from build123d import *

# Parameters (mm, degrees)
F0_W        = 15
F0_H        = 15
F0_W_2      = 7
F0_H_2      = 7
F1_DEPTH    = 4
F2_W        = 7
F2_H        = 7
F3_DEPTH    = 4
F3_TAPER    = 5
F4_W        = 7
F4_H        = 4
F5_DEPTH    = 25
F6_W        = 7
F6_H        = 4
F7_DEPTH    = 25
F8_T1_DEPTH = 37.1662479036
F9_R        = 2.5


# Not quite as in the source:
# - a fillet or chamfer that OpenCascade refuses, or shapes differently, is made with other operations: its cross-section is extruded or revolved along the edge and cut away or added


with BuildPart() as f1:
    # F0 (on Top) → F1 (new body)
    with BuildSketch(Plane.XY):
        Rectangle(F0_W, F0_H)
        Rectangle(F0_W_2, F0_H_2, mode=Mode.SUBTRACT)
        Rectangle(F0_W_2, F0_H_2)
    extrude(amount=F1_DEPTH)

    # F2 (on face) → F3 (cut)
    with BuildSketch(Plane.XY.offset(4)):
        Rectangle(F2_W, F2_H)
    extrude(amount=-F3_DEPTH, taper=F3_TAPER, mode=Mode.SUBTRACT)

    # F4 (on face) → F5 (join)
    with BuildSketch(Plane.YZ.offset(7.5)):
        with Locations((0, 2)):
            Rectangle(F4_W, F4_H)
    extrude(amount=F5_DEPTH)

    # F6 (on face) → F7 (join)
    with BuildSketch(Plane(origin=(-7.5, 0, 0), x_dir=(0, -1, 0), z_dir=(-1, 0, 0))):
        with Locations((0, 2)):
            Rectangle(F6_W, F6_H)
    extrude(amount=F7_DEPTH)

    # F8: fillet of radius 7.5 on 4 edges, made by hand

    # F8_s2 → F8_t1 (cut)
    with BuildSketch(Plane.XY.offset(-16.5831239518)):
        with BuildLine():
            ThreePointArc((-0.8667504193, 7.5), (-4.7397337655, 6.4226162893), (-7.5, 3.5))
            Line((-7.5, 3.5), (-7.5, 7.5))
            Line((-7.5, 7.5), (-0.8667504193, 7.5))
        make_face()
        with BuildLine():
            ThreePointArc((7.5, 3.5), (4.7397337655, 6.4226162893), (0.8667504193, 7.5))
            Line((0.8667504193, 7.5), (7.5, 7.5))
            Line((7.5, 7.5), (7.5, 3.5))
        make_face()
        with BuildLine():
            ThreePointArc((7.5, -3.5), (4.7397337655, -6.4226162893), (0.8667504193, -7.5))
            Line((0.8667504193, -7.5), (7.5, -7.5))
            Line((7.5, -7.5), (7.5, -3.5))
        make_face()
        with BuildLine():
            ThreePointArc((-0.8667504193, -7.5), (-4.7397337655, -6.4226162893), (-7.5, -3.5))
            Line((-7.5, -3.5), (-7.5, -7.5))
            Line((-7.5, -7.5), (-0.8667504193, -7.5))
        make_face()
    extrude(amount=F8_T1_DEPTH, mode=Mode.SUBTRACT)

    # F9
    f9_edges = [f1.edges().sort_by_distance(p)[0] for p in [
        (-32.5, 0, 0),
        (-20, -3.5, 0),
        (-20, 3.5, 0),
        (20, 3.5, 0),
        (32.5, 0, 0),
        (20, -3.5, 0),
    ]]
    fillet(f9_edges, radius=F9_R)


solid = f1.part
Model file for the job. Use its own axes, mm. A direction names the side the tool comes from. Give positions to 0.01 mm unless a question says otherwise; leave off trailing zeros. Loops run counter-clockwise (first coordinate to the right, second up) from the corner with the lowest first, then second, coordinate; pieces in that order, holes last.
1) Saw through at C-C (x = 5.5). Write the cut outline in (y, z), plus the area to 3 significant figures.
2) Wall check: line 1 (Y direction, x = -11.5, z = 2.7); line 2 (Y direction, x = -3, z = 1.05); line 3 (X direction, y = 0, z = 2.15). Give the ranges that are in metal, low to high.
3) Pull direction Z, two halves, no side cores. Call faces 1 (the flat face through (32.5, 0, 3)), 2 (the cylindrical face through (-20, -3, 1)): +Z half, -Z half, draft (parallel to the pull), parting line (faces both ways), or undercut.
4) Flat gauge pins, fed straight in: pin 1 Ø1.2 at (x, z) = (24.5, 3.5) entering from -Y; pin 2 Ø1.2 at (x, z) = (-23.5, 3.5) entering from +Y; pin 3 Ø1 at (y, z) = (0.5, 1) entering from -X. Where does each tip first touch, or does it go through?
5) Tool access for faces 3 (the cylindrical face through (20, 3, 1)), 4 (the flat face through (-20, 3.5, 3)), 5 (the flat face through (-20, -3.5, 3)), 6 (the cylindrical face through (-20, 3, 1)), 7 (the flat face through (20, -3.5, 3)): list every direction of +Z, -Z, +X, -X, +Y, -Y with a clear straight run to the whole face (end or side of a thin tool).
6) Saw through at A-A (x = -22.5). Write the cut outline in (y, z).
7) Saw through at B-B (y = 6). Write the cut outline in (x, z), plus the area to 3 significant figures.
Answer block:
1. outline: (-5.9, 0) - (5.9, 0) - (5.9, 4) - (-5.9, 4) - close
1. area: 47.2 mm2
2. line 1: y = -3.5 to 3.5
2. line 2: y = -7.19 to -3.24, 3.24 to 7.19
2. line 3: x = -32.48 to -3.34, 3.34 to 32.48
3. face 1: draft
3. face 2: -Z half
4. pin 1: stops at y = -3.5
4. pin 2: stops at y = 3.5
4. pin 3: stops at x = -32.29
5. face 3: -Z, +X, +Y
5. face 4: +Z, -Z, -X, +Y
5. face 5: +Z, -Z, -X, -Y
5. face 6: -Z, -X, +Y
5. face 7: +Z, -Z, +X, -Y
6. outline: (-3.5, 2.5) arc R2.5 ccw to (-1, 0) - (1, 0) arc R2.5 ccw to (3.5, 2.5) - (3.5, 4) - (-3.5, 4) - close
7. outline: (-5.37, 0) - (5.37, 0) - (5.37, 4) - (-5.37, 4) - close
7. area: 42.9 mm2
